Geometry check sheet. Reference: the model listing, model coordinates, mm. Face numbers are marked on the shaded views. A direction names the side the tool comes from. Give positions to 0.01 mm unless a question says otherwise; leave off trailing zeros. Order: outer loops, then holes, each group sorted by start corner. A loop starts at its lowest first (then second) coordinate and runs counter-clockwise, first axis right, second up.
from build123d import *

# Parameters (mm, degrees)
PAD_DEPTH    = 6.1
POCKET_DEPTH = 2.4
SKETCH002_R  = 6.1
PAD001_DEPTH = 4.4
SKETCH003_R  = 2.45
PAD002_DEPTH = 3.7


with BuildPart() as part:
    # Sketch → Pad (new body, symmetric)
    with BuildSketch(Plane.XZ):
        Polygon((-11.6, 23.9), (-11.6, 19.6), (-16.2, 19.6), (-16.2, 17.2), (-11.6, 17.2), (-11.6, 0), (11.6, 0), (11.6, 17.2), (16.2, 17.2), (16.2, 19.6), (11.6, 19.6), (11.6, 23.9), align=None)
    extrude(amount=PAD_DEPTH, both=True)

    # Sketch001 (on Face2 of Pad) → Pocket (cut)
    with BuildSketch(Plane(origin=(0, 0, 19.6), x_dir=(-1, 0, 0), z_dir=(0, 0, 1))):
        with BuildLine():
            Line((-16.2, 0.6), (-15.114911, 0.6))
            ThreePointArc((-15.114911, -0.6), (-12.45, 0), (-15.114911, 0.6))
            Line((-16.2, -0.6), (-15.114911, -0.6))
            Line((-16.2, 0.6), (-16.2, -0.6))
        make_face()
        with BuildLine():
            Line((16.2, 0.6), (15.114911, 0.6))
            ThreePointArc((15.114911, 0.6), (12.45, 0), (15.114911, -0.6))
            Line((16.2, -0.6), (15.114911, -0.6))
            Line((16.2, 0.6), (16.2, -0.6))
        make_face()
    extrude(amount=-POCKET_DEPTH, mode=Mode.SUBTRACT)

    # Sketch002 (on Face2 of Pocket) → Pad001 (join)
    with BuildSketch(Plane(origin=(0, 0, 23.9), x_dir=(-1, 0, 0), z_dir=(0, 0, 1))):
        with Locations((-5.5, 0)):
            Circle(SKETCH002_R)
    extrude(amount=PAD001_DEPTH)

    # Sketch003 (on Face23 of Pad001) → Pad002 (join)
    with BuildSketch(Plane(origin=(0, 0, 28.3), x_dir=(-1, 0, 0), z_dir=(0, 0, 1))):
        with Locations((-5.5, 0)):
            Circle(SKETCH003_R)
    extrude(amount=PAD002_DEPTH)


solid = part.part
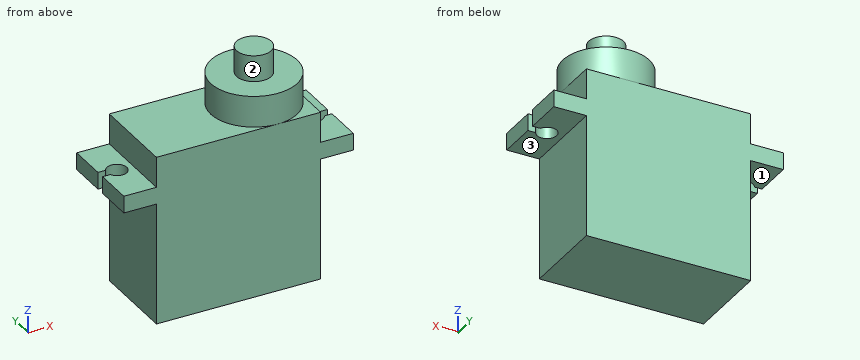
Item 1: Set-up check for the marked faces 1, 2 and 3: record each of +Z, -Z, +X, -X, +Y, -Y from which the full face is reachable in a straight line by a thin tool's end or side.
Reported:
face 1: -Z, -X, +Y, -Y
face 2: +Z
face 3: -Z, +X, +Y, -Y
Item 2: Sectioned sample at A-A (x = -13.85). Enter the section's corners in (y, z).
Reported:
outline: (-6.1, 17.2) - (-1.4, 17.2) - (-1.4, 19.6) - (-6.1, 19.6) - close; (1.4, 17.2) - (6.1, 17.2) - (6.1, 19.6) - (1.4, 19.6) - close
Item 3: Gauge pin test, flat ends, axial feed: pin 1 (1.5 mm diameter, centred on y = -2.5, z = 28.5, fed in from +X); pin 2 (3 mm diameter, centred on y = -3.5, z = 8.5, fed in from -X); pin 3 (1.4 mm diameter, centred on x = 14, y = -2.5, fed in from +Z). Record the tip position at first contact, or that the pin passes through.
Reported:
pin 1: stops at x = 11.34
pin 2: stops at x = -11.6
pin 3: stops at z = 19.6
Item 4: Sectioned sample at D-D (z = 14). Enter the section's corners in (x, y).
Reported:
outline: (-11.6, -6.1) - (11.6, -6.1) - (11.6, 6.1) - (-11.6, 6.1) - close
Item 5: Sectioned sample at B-B (x = 4). Enter the section's corners in (y, z).
Reported:
outline: (-6.1, 0) - (6.1, 0) - (6.1, 23.9) - (5.91, 23.9) - (5.91, 28.3) - (1.94, 28.3) - (1.94, 32) - (-1.94, 32) - (-1.94, 28.3) - (-5.91, 28.3) - (-5.91, 23.9) - (-6.1, 23.9) - close
Item 6: Sectioned sample at C-C (y = 4.5). Enter the section's corners in (x, z).
Reported:
outline: (-16.2, 17.2) - (-11.6, 17.2) - (-11.6, 0) - (11.6, 0) - (11.6, 17.2) - (16.2, 17.2) - (16.2, 19.6) - (11.6, 19.6) - (11.6, 23.9) - (9.62, 23.9) - (9.62, 28.3) - (1.38, 28.3) - (1.38, 23.9) - (-11.6, 23.9) - (-11.6, 19.6) - (-16.2, 19.6) - close
Item 7: Scan lines: L1, parallel to Y at x = -13.85, z = 18.2; L2, parallel to X at y = 1.25, z = 19; L3, parallel to Z at x = -5.5, y = 0.75. Record each from-to range of solid material in increasing order.
Reported:
L1: y = -6.1 to -1.4, 1.4 to 6.1
L2: x = -16.2 to -14.48, -13.22 to 13.22, 14.48 to 16.2
L3: z = 0 to 23.9
